Verification items for the finished model (mm, model axes). Face numbers are marked on the shaded views. Coordinates: 2 decimals unless noted, no trailing zeros. Write each loop counter-clockwise with the first axis right and the second up, starting at its lowest first coordinate (ties: lowest second). Pieces come first, ordered by that corner, then holes. Notation, with made-up numbers: (52, -24.5) -> (92, -24.5) arc R32 ccw to (92, 4.5) -> close; hole circle Ø3 at (-9, 59). An arc over 180 degrees is marked (long way). Use CSV: the item, a comma, the result in double quotes.
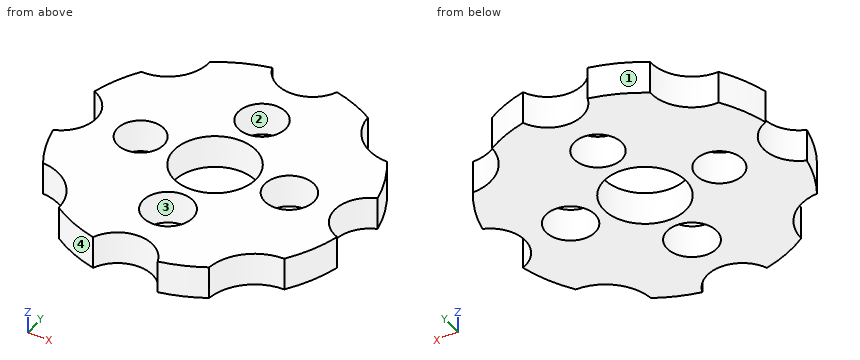
```python
from build123d import *

# Parameters (mm, degrees)
F0_R     = 9.616889
F0_R_2   = 8.985077
F0_R_3   = 15.863609
F0_R_4   = 9.540201
F0_R_5   = 9.211903
F1_DEPTH = 6.35


with BuildPart() as f1:
    # F0 (on Top) → F1 (new body, symmetric)
    with BuildSketch(Plane.XY):
        with BuildLine():
            ThreePointArc((55.750749, -12.350976), (46.941552, 0.294295), (55.591506, 13.049024))
            ThreePointArc((55.591506, 13.049024), (52.341403, 22.826962), (47.387013, 31.861632))
            ThreePointArc((47.387013, 31.861632), (34.764291, 36.976449), (28.881476, 49.260054))
            ThreePointArc((28.881476, 49.260054), (21.028254, 53.089595), (12.682723, 55.676217))
            ThreePointArc((12.682723, 55.676217), (0, 46.99), (-12.682723, 55.676217))
            ThreePointArc((-12.682723, 55.676217), (-22.699262, 52.396909), (-31.942484, 47.33255))
            ThreePointArc((-31.942484, 47.33255), (-36.40324, 35.364075), (-48.237544, 30.558664))
            ThreePointArc((-48.237544, 30.558664), (-52.651044, 22.103398), (-55.595625, 13.031466))
            ThreePointArc((-55.595625, 13.031466), (-46.989078, 0.294335), (-55.754511, -12.333979))
            ThreePointArc((-55.754511, -12.333979), (-52.979063, -21.305198), (-48.770789, -29.700214))
            ThreePointArc((-48.770789, -29.700214), (-36.390639, -35.377041), (-31.065705, -47.912572))
            ThreePointArc((-31.065705, -47.912572), (-22.21598, -52.603639), (-12.682723, -55.676217))
            ThreePointArc((-12.682723, -55.676217), (0, -46.99), (12.682723, -55.676217))
            ThreePointArc((12.682723, -55.676217), (21.002263, -53.099882), (28.833236, -49.288306))
            ThreePointArc((28.833236, -49.288306), (34.727362, -37.011133), (47.354571, -31.90983))
            ThreePointArc((47.354571, -31.90983), (52.47203, -22.525068), (55.750749, -12.350976))
        make_face()
        with Locations((0, -29.21)):
            Circle(F0_R, mode=Mode.SUBTRACT)
        with Locations((-29.21, 0)):
            Circle(F0_R_2, mode=Mode.SUBTRACT)
        Circle(F0_R_3, mode=Mode.SUBTRACT)
        with Locations((29.21, 0)):
            Circle(F0_R_4, mode=Mode.SUBTRACT)
        with Locations((0, 29.21)):
            Circle(F0_R_5, mode=Mode.SUBTRACT)
    extrude(amount=F1_DEPTH, both=True)


solid = f1.part
```
1) Gauge pin test, flat ends, axial feed: pin 1 (6 mm diameter, centred on x = 8, z = 4, fed in from -Y); pin 2 (3 mm diameter, centred on y = 16, z = -0.5, fed in from -X); pin 3 (1 mm diameter, centred on x = -39, z = 1.5, fed in from +Y). Record the tip position at first contact, or that the pin passes through.
Return value:
pin 1,"y = -52.59"
pin 2,"x = -55.23"
pin 3,"y = 33.55"
2) Cross-section at B-B (y = 7). Record the boundary of the cut face in (x, z).
Return value:
outline,"(-48.71, -6.35) -> (-34.84, -6.35) -> (-34.84, 6.35) -> (-48.71, 6.35) -> close; (-23.58, -6.35) -> (-14.24, -6.35) -> (-14.24, 6.35) -> (-23.58, 6.35) -> close; (14.24, -6.35) -> (22.73, -6.35) -> (22.73, 6.35) -> (14.24, 6.35) -> close; (35.69, -6.35) -> (48.66, -6.35) -> (48.66, 6.35) -> (35.69, 6.35) -> close"
3) Cross-section at A-A (x = 0). Record the boundary of the cut face in (y, z), plus the area to 3 significant figures.
Return value:
outline,"(-46.99, -6.35) -> (-38.83, -6.35) -> (-38.83, 6.35) -> (-46.99, 6.35) -> close; (-19.59, -6.35) -> (-15.86, -6.35) -> (-15.86, 6.35) -> (-19.59, 6.35) -> close; (15.86, -6.35) -> (20, -6.35) -> (20, 6.35) -> (15.86, 6.35) -> close; (38.42, -6.35) -> (46.99, -6.35) -> (46.99, 6.35) -> (38.42, 6.35) -> close"
area,"312 mm2"
4) Cross-section at C-C (x = 30.5). Record the boundary of the cut face in (y, z), plus the area to 3 significant figures.
Return value:
outline,"(-42.88, -6.35) -> (-9.45, -6.35) -> (-9.45, 6.35) -> (-42.88, 6.35) -> close; (9.45, -6.35) -> (42.94, -6.35) -> (42.94, 6.35) -> (9.45, 6.35) -> close"
area,"850 mm2"
5) Mould release check, pull along Y, two halves, no side actions. Record for the marked faces 1, 2, 3 and 4: released by +Y, released by -Y, zero draft, split by the parting line, or undercut.
Return value:
face 1,"released by +Y"
face 2,"undercut"
face 3,"undercut"
face 4,"released by -Y"
6) Cross-section at D-D (y = 29.21). Record the boundary of the cut face in (x, z), plus the area to 3 significant figures.
Return value:
outline,"(-49.07, -6.35) -> (-9.21, -6.35) -> (-9.21, 6.35) -> (-49.07, 6.35) -> close; (9.21, -6.35) -> (49.07, -6.35) -> (49.07, 6.35) -> (9.21, 6.35) -> close"
area,"1,010 mm2"
7) Scan lines: L1, parallel to Y at x = 0, z = -0.75; L2, parallel to X at y = -4.5, z = 1.75; L3, parallel to X at y = 1.5, z = 4. Record each from-to range of solid material in increasing order.
Return value:
L1,"-46.99 to -38.83, -19.59 to -15.86, 15.86 to 20, 38.42 to 46.99"
L2,"-47.89 to -36.99, -21.43 to -15.21, 15.21 to 20.8, 37.62 to 47.85"
L3,"-47.04 to -38.07, -20.35 to -15.79, 15.79 to 19.79, 38.63 to 46.99"
